from build123d import *

# Parameters (mm, degrees)
F1_DEPTH = 30.1625
F0_R     = 26.9875
F2_DEPTH = 38.1
F3_R     = 8.73125
F4_DEPTH = 25.4
F5_R     = 8.73125
F6_DEPTH = 25.4
F8_R     = 2.38125
F9_DEPTH = 25.4


with BuildPart() as f1:
    # F0 (on Front) → F1 (new body, symmetric)
    with BuildSketch(Plane.XZ):
        with BuildLine():
            Line((-88.9, 15.875), (-88.9, 0))
            Line((-88.9, 0), (-44.45, 0))
            ThreePointArc((-44.45, 0), (-43.520064, 2.245064), (-41.275, 3.175))
            Line((-41.275, 3.175), (41.275, 3.175))
            ThreePointArc((41.275, 3.175), (43.520064, 2.245064), (44.45, 0))
            Line((44.45, 0), (88.9, 0))
            Line((88.9, 0), (88.9, 15.875))
            ThreePointArc((88.9, 15.875), (87.040128, 20.365128), (82.55, 22.225))
            Line((82.55, 22.225), (47.625, 22.225))
            ThreePointArc((47.625, 22.225), (40.889808, 25.014808), (38.1, 31.75))
            Line((38.1, 31.75), (38.1, 76.2))
            ThreePointArc((38.1, 76.2), (0, 38.1), (-38.1, 76.2))
            Line((-38.1, 76.2), (-38.1, 31.75))
            ThreePointArc((-38.1, 31.75), (-40.889808, 25.014808), (-47.625, 22.225))
            Line((-47.625, 22.225), (-82.55, 22.225))
            ThreePointArc((-82.55, 22.225), (-87.040128, 20.365128), (-88.9, 15.875))
        make_face()
    extrude(amount=F1_DEPTH, both=True)

    # F0 (on Front) → F2 (join, symmetric)
    with BuildSketch(Plane.XZ):
        with BuildLine():
            ThreePointArc((38.1, 76.2), (0, 114.3), (-38.1, 76.2))
            ThreePointArc((-38.1, 76.2), (0, 38.1), (38.1, 76.2))
        make_face()
        with Locations((0, 76.2)):
            Circle(F0_R, mode=Mode.SUBTRACT)
    extrude(amount=F2_DEPTH, both=True)

    # F3 (on face) → F4 (cut)
    with BuildSketch(Plane.XY.offset(22.225)):
        with Locations((72.782576, 0)):
            Circle(F3_R)
    extrude(amount=-F4_DEPTH, mode=Mode.SUBTRACT)

    # F5 (on face) → F6 (cut)
    with BuildSketch(Plane.XY.offset(22.225)):
        with Locations((-73.331527, 0)):
            Circle(F5_R)
    extrude(amount=-F6_DEPTH, mode=Mode.SUBTRACT)

    # F8 (on offset) → F9 (cut)
    with BuildSketch(Plane.XY.offset(114.3)):
        Circle(F8_R)
    extrude(amount=-F9_DEPTH, mode=Mode.SUBTRACT)


solid = f1.part
Could you check a few things on this model? Use its own coordinates, in mm. A direction names the side the tool comes from. Round coordinates to 2 decimals unless told otherwise and drop trailing zeros. Loops run counter-clockwise (first coordinate to the right, second up) from the corner with the lowest first, then second, coordinate; pieces in that order, holes last. Notation, with made-up numbers: (69, -38) - (77, -38) arc R18 ccw to (77, -4) - close; hole circle Ø7 at (59.25, 37.5). An arc over 180 degrees is marked (long way). Write item = value, one per line.
1) Imagine slicing it at A-A (x = 0). Please give me the cut outline in (y, z) (1 decimal).
Computed:
outline = (-38.1, 38.1) - (-30.2, 38.1) - (-30.2, 3.2) - (30.2, 3.2) - (30.2, 38.1) - (38.1, 38.1) - (38.1, 49.2) - (-38.1, 49.2) - close; (-38.1, 103.2) - (-2.4, 103.2) - (-2.4, 114.3) - (-38.1, 114.3) - close; (2.4, 103.2) - (38.1, 103.2) - (38.1, 114.3) - (2.4, 114.3) - close
2) If we mould it in two halves opening along Y, with no side actions, what happens to faces 4 (the flat face through (-38.1, 0, 54)), 5 (the cylindrical face through (80.85, -3.34, 11.27)), 6 (the flat face through (-1, 30.162, 13))? For each: pulls with the +Y half, pulls with the -Y half, needs draft (parallel to the pull), parting line crosses it, or undercut.
Computed:
face_4 = needs draft
face_5 = undercut
face_6 = pulls with the +Y half
3) Imagine slicing it at B-B (y = 0). Give the number of separate pieces and of enclosed holes in the cut face, and give its area (3 significant figures).
Computed:
separate_pieces = 3
enclosed_holes = 0
area = 6,970 mm2
4) On a 3-axis mill with a long thin cutter (end or side, diameter ignored), from which of +Z, -Z, +X, -X, +Y, -Y can I reach the whole of each face in a straight line? I mean faces 1 (the flat face through (61, 0, 22.225)), 2 (the flat face through (-1, 0, 3.175)), 3 (the cylindrical face through (-1.89, -1.45, 108.77)). Say none if no direction works.
Computed:
face_1 = +Z, +X, +Y, -Y
face_2 = -Z, +Y, -Y
face_3 = +Z
5) Imagine slicing it at C-C (z = 56.5). Please give me the cut outline in (x, y).
Computed:
outline = (-38.1, -30.16) - (-32.61, -30.16) - (-32.61, -38.1) - (-18.45, -38.1) - (-18.45, 38.1) - (-32.61, 38.1) - (-32.61, 30.16) - (-38.1, 30.16) - close; (18.45, -38.1) - (32.61, -38.1) - (32.61, -30.16) - (38.1, -30.16) - (38.1, 30.16) - (32.61, 30.16) - (32.61, 38.1) - (18.45, 38.1) - close
6) I need wall thicknesses on line 1 along Y through (x, z) = (0, 111.75); line 2 along X through (y, z) = (8, 16.5); line 3 along Y through (x, z) = (64, 14.5). Which ranges of each line are inside material? Lowest first, please. Write a range as from..to.
Computed:
line_1 = -38.1..-2.38, 2.38..38.1
line_2 = -88.87..-76.83, -69.83..69.28, 76.28..88.87
line_3 = -30.16..30.16
7) I'm going to push flat-ended pins straight in: P1, Ø13.5, axis at y = 13.5, z = 61.5, coming from the +X side; P2, Ø1, axis at x = -55, z = 22.5, coming from the -Y side; P3, Ø22.5, axis at x = 72.78, y = 0, coming from the +Z side (3 decimals). Where does each tip first touch, or does it pass through?
Computed:
P1 = 38.1
P2 = -30.16
P3 = 22.225
